Can you work these out from the drawing? Everything is in mm from the part's minimum corner. Give positions to 0.01 mm unless a question says otherwise; leave off trailing zeros. Order: outer loops, then holes, each group sorted by start corner. A loop starts at its lowest first (then second) coordinate and runs counter-clockwise, first axis right, second up. Notation, with made-up numbers: (-7.75, 8.5) -> (23.25, 8.5) arc R13 cw to (23.25, 13.5) -> close; hole circle Ø1 at (35, -15.75). An arc over 180 degrees is marked (long way). One line per item, written item: value.
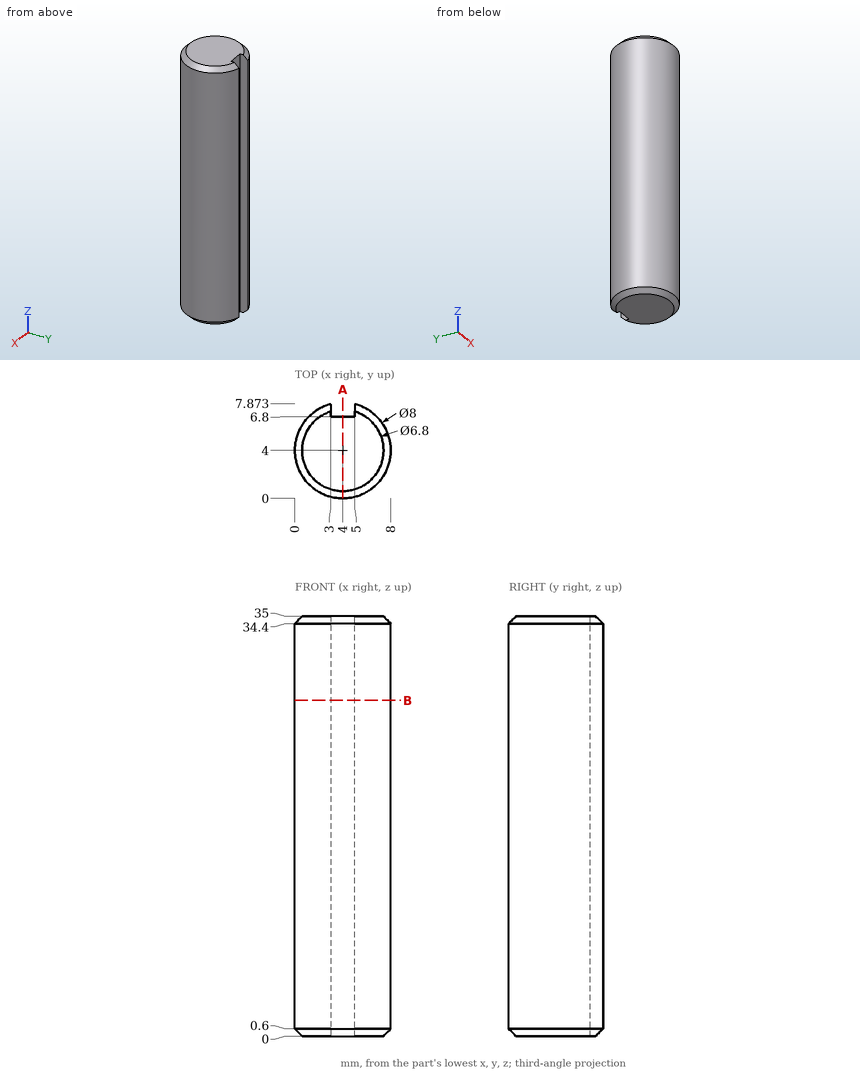
1) Suppose I cut it at B-B, the plane z = 28. Write out the boundary of the cut face in (x, y), then the cut area to 4 significant figures.
Answer below:
outline: (3, 6.8) -> (3, 7.87) arc R4 ccw (long way) to (5, 7.87) -> (5, 6.8) -> close
area: 47.95 mm2
2) Suppose I cut it at A-A, the plane x = 4. Write out the boundary of the cut face in (y, z).
Answer below:
outline: (0, 0.6) -> (0.6, 0) -> (6.8, 0) -> (6.8, 35) -> (0.6, 35) -> (0, 34.4) -> close
3) If I drill on line 1 along Y through (x, z) = (4, 5); line 2 along X through (y, z) = (4.25, 20.5); line 3 along X through (y, z) = (0.75, 4.5), over which ranges is the centre line in solid material (lowest first)?
Answer below:
line 1: y = 0 to 6.8
line 2: x = 0.01 to 7.99
line 3: x = 1.67 to 6.33
4) For P1, Ø1.2, axis at y = 7.5, z = 12, coming from the -X side (3 decimals); P2, Ø3, axis at x = 6.5, z = 8.5, coming from the -Y side; P3, Ø0.5, axis at y = 7, z = 11.5, coming from the +X side, each with a flat end and sliding along its axis, tell me the tip position at first contact or that it passes through.
Answer below:
P1: stops at x = 1.245
P2: stops at y = 0.13
P3: stops at x = 6.9
